Check sheet for the modelled part. Datum: model origin and axes. Units: mm. Face numbers are marked on the shaded views. Give positions to 0.01 mm unless a question says otherwise; leave off trailing zeros. Loops run counter-clockwise (first coordinate to the right, second up) from the corner with the lowest first, then second, coordinate; pieces in that order, holes last. Notation, with made-up numbers: (64.25, 14) -> (70.25, 14) arc R16 cw to (70.25, 28) -> close; hole circle Ø9 at (46, -39.75). An arc over 180 degrees is marked (long way). Answer as CSV lines item,"result". Start each with the question number.
(1) Section check A-A on z = 2. Enter the section's corners in (x, y).
(2) Section check C-C on z = 6.75. Enter the section's corners in (x, y).
(3) Release check for a two-part mould opening along Y. For the marked faces 1, 2 and 3 record: pulls with the +Y half, pulls with the -Y half, needs draft (parallel to the pull), parting line crosses it, or undercut.
(4) Gauge pin test, flat ends, axial feed: pin 1 Ø2.5 at (x, y) = (1, -0.5) entering from -Z; pin 2 Ø4 at (x, y) = (0, 0) entering from +Z; pin 3 Ø4 at (x, z) = (-4, 4) entering from -Y; pin 4 Ø2.5 at (x, y) = (0, 0) entering from -Z. Record the tip position at first contact, or that the pin passes through.
(5) Material ranges on line 1 (X direction, y = 0, z = 6.1); line 2 (Y direction, x = 2, z = 9.25); line 3 (X direction, y = -1, z = 6), recorded low to high. Write a range as from..to.
(6) Section check B-B on y = 4.25. Enter the section's corners in (x, z), plus the area to 3 significant figures.
(7) Section check D-D on y = 8.5. Enter the section's corners in (x, z).
from build123d import *

# Parameters (mm, degrees)
SKETCH1_R           = 1.5
BOSS_EXTRUDE3_DEPTH = 8
SKETCH2_R           = 5
BOSS_EXTRUDE4_DEPTH = 3
CUT_EXTRUDE1_DEPTH  = 4
SKETCH5_R           = 2.4
CUT_EXTRUDE2_DEPTH  = 4
CHAMFER1_SIZE       = 0.8


with BuildPart() as part:
    # Sketch1 → Boss-Extrude3 (new body)
    with BuildSketch(Plane.XY):
        with BuildLine():
            Line((-3.2, 3.841874542), (-1.678558667, 13.728155368))
            ThreePointArc((-1.678558667, 13.728155368), (-1.172681412, 14.638471135), (-0.196011829, 15))
            Line((-0.196011829, 15), (0.196011829, 15))
            ThreePointArc((0.196011829, 15), (1.172681412, 14.638471135), (1.678558667, 13.728155368))
            Line((1.678558667, 13.728155368), (3.2, 3.841874542))
            ThreePointArc((3.2, 3.841874542), (0, -5), (-3.2, 3.841874542))
        make_face()
        Circle(SKETCH1_R, mode=Mode.SUBTRACT)
    extrude(amount=BOSS_EXTRUDE3_DEPTH)

    # Sketch2 → Boss-Extrude4 (add)
    with BuildSketch(Plane.XY.offset(8)):
        with Locations(Location((0, 0, 0), (0, 0, 129.7918195))):
            Circle(SKETCH2_R)
    extrude(amount=BOSS_EXTRUDE4_DEPTH)

    # Sketch4 → Cut-Extrude1 (cut)
    with BuildSketch(Plane.XY.offset(11)):
        Polygon((-2.992716352, 0.588344146), (-2.610587457, 0.864484315), (-2.752379426, 1.314118525), (-2.313582545, 1.48655165), (-2.339100377, 1.957322004), (-1.871206732, 2.015213479), (-1.778847049, 2.477539743), (-1.311256119, 2.417252033), (-1.106822219, 2.842084548), (-0.668914462, 2.667405751), (-0.365251678, 3.028050728), (0.015457551, 2.749956557), (0.399268969, 3.023753345), (0.69885831, 2.659717478), (1.138702078, 2.829462418), (1.33834723, 2.402358568), (1.806586348, 2.457385962), (1.893742872, 1.994050635), (2.360956154, 1.930902908), (2.330147685, 1.460449166), (2.766978401, 1.283094123), (2.620140749, 0.835082305), (2.999141219, 0.554663816), (2.745500733, 0.157244152), (3.042856964, -0.208618059), (2.698350809, -0.53047423), (2.895378816, -0.958791695), (2.48165358, -1.184860965), (2.565973368, -1.648720921), (2.10902493, -1.764798528), (2.075338376, -2.235054949), (1.603878487, -2.233847309), (1.454302241, -2.680952254), (0.99795446, -2.562535248), (0.741886949, -2.95839547), (0.329325284, -2.730209673), (-0.01714383, -3.049951818), (-0.359996611, -2.726334983), (-0.775097398, -2.949868476), (-1.026698595, -2.55115464), (-1.484348746, -2.664434049), (-1.62888933, -2.215675868), (-2.100333004, -2.211583431), (-2.128730958, -1.740978032), (-2.584345614, -1.619770893), (-2.494816591, -1.156888144), (-2.905974285, -0.926182193), (-2.704143722, -0.500106719), (-3.045009904, -0.174398059), (-2.743559558, 0.18809825), align=None)
    extrude(amount=-CUT_EXTRUDE1_DEPTH, mode=Mode.SUBTRACT)

    # Sketch5 → Cut-Extrude2 (cut)
    with BuildSketch(Plane(origin=(0, 0, 0), x_dir=(-1, 0, 0), z_dir=(0, 0, -1))):
        Circle(SKETCH5_R)
    extrude(amount=-CUT_EXTRUDE2_DEPTH, mode=Mode.SUBTRACT)

    # Chamfer1
    chamfer1_edges = [part.edges().sort_by_distance(p)[0] for p in [
        (2.4, 0, 0),
        (-2.439279334, 8.785014955, 0),
        (-1.172681412, 14.638471135, 0),
        (0, 15, 0),
        (1.172681412, 14.638471135, 0),
        (2.439279334, 8.785014955, 0),
        (0, -5, 0),
    ]]
    chamfer(chamfer1_edges, length=CHAMFER1_SIZE)


solid = part.part
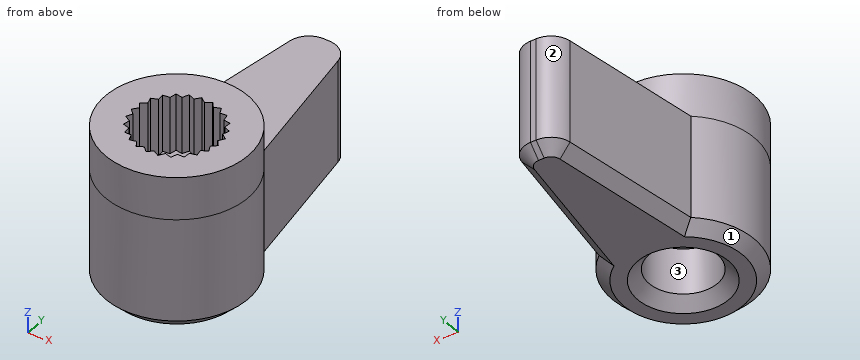
Working result:
1,outline,"(-3.2, 3.84) arc R5 ccw (long way) to (3.2, 3.84) -> (1.68, 13.73) arc R1.5 ccw to (0.2, 15) -> (-0.2, 15) arc R1.5 ccw to (-1.68, 13.73) -> close; hole circle Ø4.8 at (0, 0)"
2,outline,"(-3.2, 3.84) arc R5 ccw (long way) to (3.2, 3.84) -> (1.68, 13.73) arc R1.5 ccw to (0.2, 15) -> (-0.2, 15) arc R1.5 ccw to (-1.68, 13.73) -> close; hole circle Ø3 at (0, 0)"
3,face 1,"parting line crosses it"
3,face 2,"pulls with the +Y half"
3,face 3,"undercut"
4,pin 1,"stops at z = 4"
4,pin 2,"stops at z = 7"
4,pin 3,"stops at y = -4.58"
4,pin 4,"passes through"
5,line 1,"x = -5..-1.5, 1.5..5"
5,line 2,"y = -4.58..-2.23, 1.98..4.58"
5,line 3,"x = -4.9..-1.12, 1.12..4.9"
6,outline,"(-3.14, 0.8) -> (-2.33, 0) -> (2.33, 0) -> (3.14, 0.8) -> (3.14, 8) -> (2.63, 8) -> (2.63, 11) -> (-2.63, 11) -> (-2.63, 8) -> (-3.14, 8) -> close"
6,area,"65.4 mm^2"
7,outline,"(-2.48, 0.8) -> (-1.67, 0) -> (1.67, 0) -> (2.48, 0.8) -> (2.48, 8) -> (-2.48, 8) -> close"
